Geometry check sheet. Reference: the model listing, model coordinates, mm. A direction names the side the tool comes from. Round coordinates to 2 decimals unless told otherwise and drop trailing zeros. Order: outer loops, then holes, each group sorted by start corner. A loop starts at its lowest first (then second) coordinate and runs counter-clockwise, first axis right, second up. Notation, with made-up numbers: (84, 70) - (129, 70) arc R17 cw to (129, 79) - close; hole circle Ø11 at (-25, 50.25). An arc over 180 degrees is marked (long way). Return JSON: item names as keys, results as strings. Group by question number.
Q1. Tool access check on faces 1 (the conical face through (-137.83, -1.01, 22.09)), 2 (the flat face through (-131.714, 0, 23)). Record the directions out of +Z, -Z, +X, -X, +Y, -Y that give a thin tool (end or side, any length) a straight path to the whole face; none if there is none.
Q2. Material ranges on line 1 along Z through (x, y) = (-134, 0); line 2 along Y through (x, z) = (-142.75, 29); line 3 along Y through (x, z) = (-134.75, 26.75), recorded low to high.
Q3. Draft check along Y on faces 3 (the cylindrical face through (-135.33, -0.089, 27.333)), 4 (the flat face through (-133.238, 2, 28)), 5 (the cylindrical face through (-132.47, -4.69, 22.31)), 6 (the conical face through (-139.13, -0.1, 27.58)). Enter one of: pulls with the +Y half, pulls with the -Y half, needs draft (parallel to the pull), parting line crosses it, or undercut.
Q4. Gauge pin test, flat ends, axial feed: pin 1 Ø5 at (y, z) = (-5, 28.5) entering from +X; pin 2 Ø2.5 at (y, z) = (0, 25.3) entering from -X (3 decimals); pin 3 Ø3 at (x, z) = (-135, 29.5) entering from +Y; pin 4 Ø4 at (x, y) = (-139.5, -3) entering from +Z. Record the tip position at first contact, or that the pin passes through.
Q5. Sectioned sample at B-B, the plane x = -135. Record the cut outline in (y, z) (3 decimals), then the cut area to 3 significant figures.
Q6. Sectioned sample at C-C, the plane x = -138.5. Record the cut outline in (y, z), then the cut area to 3 significant figures.
Q7. Sectioned sample at A-A, the plane y = 0. Record the cut outline in (x, z), then the cut area to 3 significant figures.
```python
from build123d import *


with BuildPart() as f1:
    # F0 (on Front) → F1 (revolve)
    with BuildSketch(Plane.XZ):
        with BuildLine():
            Line((-131.713825, 19.739976), (-131.713825, 23.270576))
            Line((-131.713825, 23.270576), (-138.847012, 23.270576))
            Line((-138.847012, 23.270576), (-143.371043, 19.337896))
            ThreePointArc((-143.371043, 19.337896), (-143.059541, 18.498054), (-142.271226, 18.072701))
            Line((-142.271226, 18.072701), (-137.606625, 22.127576))
            Line((-137.606625, 22.127576), (-133.237825, 22.127576))
            Line((-133.237825, 22.127576), (-133.237825, 19.739976))
            Line((-133.237825, 19.739976), (-131.713825, 19.739976))
        make_face()
    revolve(axis=Axis((-144.413825, 0, 25.302576), (-1, 0, 0)))


solid = f1.part
```
Reply:
{
 "1": {"face 1": "none", "face 2": "+Z, -Z, +X, +Y, -Y"},
 "2": {"line 1": "22.13 to 23.27, 27.33 to 28.48", "line 2": "-6.02 to -3.97, 3.97 to 6.02", "line 3": "-2.83 to -1.43, 1.43 to 2.83"},
 "3": {"face 3": "undercut", "face 4": "needs draft", "face 5": "parting line crosses it", "face 6": "undercut"},
 "4": {"pin 1": "x = -131.71", "pin 2": "through", "pin 3": "y = 1.67", "pin 4": "z = 31.33"},
 "5": {"outline": "circle Ø6.35 at (0, 25.303); hole circle Ø4.064 at (0, 25.303)", "area": "18.7 mm^2"},
 "6": {"outline": "circle Ø7.9 at (0, 25.3); hole circle Ø4.06 at (0, 25.3)", "area": "36.1 mm^2"},
 "7": {"outline": "(-143.37, 19.34) arc R1.27 ccw to (-142.27, 18.07) - (-137.61, 22.13) - (-133.24, 22.13) - (-133.24, 19.74) - (-131.71, 19.74) - (-131.71, 23.27) - (-138.85, 23.27) - close; (-143.37, 31.27) - (-138.85, 27.33) - (-131.71, 27.33) - (-131.71, 30.87) - (-133.24, 30.87) - (-133.24, 28.48) - (-137.61, 28.48) - (-142.27, 32.53) arc R1.27 ccw to start", "area": "43.3 mm^2"}
}
